```python
from build123d import *

# Parameters (mm, degrees)
F0_W          = 10.2
F0_H          = 7
F1_DEPTH      = 1.5
F2_W          = 11.2
F2_H          = 46
F3_DEPTH      = 25
F4_W          = 1.5
F4_H          = 70.9369339572
F5_DEPTH      = 10.5
F6_W          = 45.52
F6_H          = 10.5
F6_R          = 1.3
F6_W_2        = 3.43
F6_W_3        = 6.1469339572
F7_DEPTH      = 25
F9_DEPTH      = 0.5
F10_T4_DEPTH  = 23.6102213202
F10_T10_DEPTH = 23.6102213202
F11_W         = 18.4
F11_H         = 1.5
F12_DEPTH     = 11.5
F14_DEPTH     = 1.5


# Not quite as in the source:
# - a fillet or chamfer that OpenCascade refuses, or shapes differently, is made with other operations: its cross-section is extruded or revolved along the edge and cut away or added


with BuildPart() as f1:
    # F0 (on Top) → F1 (new body)
    with BuildSketch(Plane.XY):
        Polygon((12.9583973216, 44.6379526287), (-5.4416026784, 44.6379526287), (-5.4416026784, -26.2989813285), (-1.3416026784, -29.5620473713), (8.8583973216, -29.5620473713), (12.9583973216, -26.2989813285), align=None)
        with Locations((3.7583973216, -33.0620473713)):
            Rectangle(F0_W, F0_H)
    extrude(amount=F1_DEPTH)

    # F2 (on face) → F3 (cut)
    with BuildSketch(Plane.XY.offset(1.5)):
        with Locations((3.3583973216, 9.8879526287)):
            Rectangle(F2_W, F2_H)
    extrude(amount=-F3_DEPTH, mode=Mode.SUBTRACT)

    # F4 (on face) → F5 (join)
    with BuildSketch(Plane(origin=(0, 0, 0), x_dir=(1, 0, 0), z_dir=(0, 0, -1))):
        with Locations((-4.6916026784, -9.1694856501)):
            Rectangle(F4_W, F4_H)
    extrude(amount=F5_DEPTH)

    # F6 (on face) → F7 (cut)
    with BuildSketch(Plane.YZ.offset(-3.9416026784)):
        with Locations((10.5479526287, -5.25)):
            Rectangle(F6_W, F6_H)
        with Locations((-16.1820473713, -7.8)):
            Circle(F6_R)
        with Locations((37.2779526287, -7.8)):
            Circle(F6_R)
        with Locations((42.9229526287, -5.25)):
            Rectangle(F6_W_2, F6_H)
        with Locations((-23.2255143499, -5.25)):
            Rectangle(F6_W_3, F6_H)
    extrude(amount=-F7_DEPTH, mode=Mode.SUBTRACT)

    # F8 (on face) → F9 (cut)
    with BuildSketch(Plane(origin=(0, 0, 0), x_dir=(1, 0, 0), z_dir=(0, 0, -1))):
        Polygon((-1.3416026784, 29.5620473713), (-2.5980896591, 28.5620473713), (10.1148843023, 28.5620473713), (8.8583973216, 29.5620473713), (8.8583973216, 36.5620473713), (-1.3416026784, 36.5620473713), align=None)
    extrude(amount=-F9_DEPTH, mode=Mode.SUBTRACT)

    # F10: fillet of radius 5 on 1 edges, made by hand


with BuildPart() as f10_tool2:
    # F10_s3 → F10_t4 (new body)
    with BuildSketch(Plane.YZ.offset(-8.0467133385)):
        with BuildLine():
            ThreePointArc((-30.7414968431, 0.5), (-29.6234628544, 0.3733971724), (-28.5620473713, 0))
            Line((-28.5620473713, 0), (-28.5620473713, 0.5))
            Line((-28.5620473713, 0.5), (-30.7414968431, 0.5))
        make_face()
    extrude(amount=F10_T4_DEPTH)

    split(bisect_by=Plane.YZ.offset(8.8583973216), keep=Keep.BOTTOM)

    split(bisect_by=Plane(origin=(-14.9242028331, -18.7520665571, 0), x_dir=(0, 0, 1), z_dir=(0.6227225273, 0.7824427481, 0)), keep=Keep.TOP)


with BuildPart() as f1_1:
    add(f1.part)

    # F10_t1: union F10_tool2
    add(f10_tool2.part)


with BuildPart() as f10_tool8:
    # F10_s9 → F10_t10 (new body)
    with BuildSketch(Plane.YZ.offset(-8.0467133385)):
        with BuildLine():
            ThreePointArc((-30.7414968431, 0.5), (-29.6234628544, 0.3733971724), (-28.5620473713, 0))
            Line((-28.5620473713, 0), (-28.5620473713, 0.5))
            Line((-28.5620473713, 0.5), (-30.7414968431, 0.5))
        make_face()
    extrude(amount=F10_T10_DEPTH)

    split(bisect_by=Plane(origin=(17.8390906107, -22.4145850999, 0), x_dir=(0, 0, 1), z_dir=(-0.6227225273, 0.7824427481, 0)), keep=Keep.TOP)

    split(bisect_by=Plane.YZ.offset(-1.3416026784), keep=Keep.TOP)


with BuildPart() as f1_2:
    add(f1_1.part)

    # F10_t7: union F10_tool8
    add(f10_tool8.part)

    # F11 (on face) → F12 (join)
    with BuildSketch(Plane.XY.offset(1.5)):
        with Locations((3.7583973216, 43.8879526287)):
            Rectangle(F11_W, F11_H)
    extrude(amount=F12_DEPTH)

    # F13 (on face) → F14 (cut, through all)
    with BuildSketch(Plane(origin=(0, 44.6379526287, 0), x_dir=(-1, 0, 0), z_dir=(0, 1, 0))):
        with BuildLine():
            ThreePointArc((-6.9583973216, 7.5), (-7.5441837593, 8.9142135624), (-8.9583973216, 9.5))
            ThreePointArc((-8.9583973216, 9.5), (-10.9583973216, 7.5), (-8.9583973216, 5.5))
            ThreePointArc((-8.9583973216, 5.5), (-7.5441837593, 6.0857864376), (-6.9583973216, 7.5))
        make_face()
        with BuildLine():
            Line((-8.9583973216, 9.5), (-12.9583973216, 9.5))
            Line((-12.9583973216, 9.5), (-12.9583973216, 5.5))
            Line((-12.9583973216, 5.5), (-8.9583973216, 5.5))
            ThreePointArc((-8.9583973216, 5.5), (-10.9583973216, 7.5), (-8.9583973216, 9.5))
        make_face()
    extrude(amount=-F14_DEPTH, mode=Mode.SUBTRACT)


solid = f1_2.part
```
For this review, take the finished solid that the model builds, in its own axes (mm). A direction names the side the tool comes from. Round coordinates to 2 decimals unless told otherwise and drop trailing zeros. Loops run counter-clockwise (first coordinate to the right, second up) from the corner with the lowest first, then second, coordinate; pieces in that order, holes last.
(1) We need section A-A (y = 24.5). Give the boundary of the cut face in (x, z).
Returned:
outline: (-5.44, 0) - (-2.24, 0) - (-2.24, 1.5) - (-5.44, 1.5) - close; (8.96, 0) - (12.96, 0) - (12.96, 1.5) - (8.96, 1.5) - close
(2) We need section C-C (z = -5.75). Give the boundary of the cut face in (x, y).
Returned:
outline: (-5.44, -20.15) - (-3.94, -20.15) - (-3.94, -12.21) - (-5.44, -12.21) - close; (-5.44, 33.31) - (-3.94, 33.31) - (-3.94, 41.21) - (-5.44, 41.21) - close
(3) Tool access review of faces 1 (the flat face through (-5, -20.152, -5)), 2 (the flat face through (8.958, 10, 1)), 3 (the flat face through (11, 44, 5.5)), 4 (the flat face through (-5, -12.212, -5)): name each direction out of +Z, -Z, +X, -X, +Y, -Y from which nothing blocks a thin tool from reaching the whole face with its end or side.
Returned:
face 1: -Z, +X, -X, -Y
face 2: +Z, -Z
face 3: +X, +Y, -Y
face 4: -Z, +X, -X
(4) We need section B-B (x = 1.75). Give the boundary of the cut face in (y, z).
Returned:
outline: (-36.56, 0.5) - (-30.74, 0.5) arc R5 cw to (-28.56, 0) - (-13.11, 0) - (-13.11, 1.5) - (-36.56, 1.5) - close; (32.89, 0) - (44.64, 0) - (44.64, 13) - (43.14, 13) - (43.14, 1.5) - (32.89, 1.5) - close
(5) Clearance check with flat-ended pins moving along their axes: P1, Ø1.2, axis at x = -4.5, z = -5.5, coming from the +Y side; P2, Ø1.6, axis at x = -5, z = -4, coming from the -Y side; P3, Ø1.5, axis at x = 1, z = 5.5, coming from the -Y side. State where each tip first meets the part, or that it passes through.
Returned:
P1: stops at y = 41.21
P2: stops at y = -20.15
P3: stops at y = 43.14
(6) Mouldability with a two-part tool opening along X and no side actions: class faces 5 (the flat face through (-3.942, -16, -5)), 6 (the flat face through (3, -13.112, 1)), 7 (the flat face through (4, 44, 13)) as released by +X, released by -X, zero draft, split by the parting line, or undercut.
Returned:
face 5: released by +X
face 6: undercut
face 7: zero draft
(7) Wall thickness on line 1 along Z through (x, y) = (7.75, 33); line 2 along Z through (x, y) = (6, -32); line 3 along X through (y, z) = (-19.5, -1.75): over which ranges is each line inside the solid? List them lowest first.
Returned:
line 1: z = 0 to 1.5
line 2: z = 0.5 to 1.5
line 3: x = -5.44 to -3.94
